Autodesk Fusion 360 part; units mm, degrees
sketch "Sketch1" plane through (0, 0, 0) normal (0, 0, 1) x (1, 0, 0) in component "Hot Plate Mounting Plate"
  line L0 (0, 0) -> (-182, 0) construction
  line L1 (-182, 0) -> (-182, -202) construction
  line L2 (-182, -202) -> (0, -202) construction
  line L3 (0, -202) -> (0, 0) construction
  line L4 (-91, -202) -> (-91, 0) construction
  line L5 (0, -101) -> (-182, -101) construction
  line L6 (-91, 0) -> (-13, 0)
  line L7 (-91, 0) -> (-169, 0)
  line L8 (-91, -202) -> (-13, -202)
  line L9 (-91, -202) -> (-169, -202)
  line L10 (0, -101) -> (0, -13)
  line L11 (0, -101) -> (0, -189)
  line L12 (-182, -101) -> (-182, -189)
  line L13 (-182, -101) -> (-182, -13)
  line L14 (-182, -13) -> (0, -13) construction
  line L15 (0, -189) -> (-182, -189) construction
  line L16 (-13, -202) -> (-13, 0) construction
  line L17 (-169, 0) -> (-169, -202) construction
  line L18 (0, -189) -> (-13, -189)
  line L19 (-13, -202) -> (-13, -189)
  line L20 (-169, -202) -> (-169, -189)
  line L21 (-182, -189) -> (-169, -189)
  line L22 (0, -13) -> (-13, -13)
  line L23 (-13, 0) -> (-13, -13)
  line L24 (-169, 0) -> (-169, -13)
  line L25 (-182, -13) -> (-169, -13)
  dimension "d1" = 182
  dimension "d2" = 202
  dimension "d3" = 78
  dimension "d4" = 78
  dimension "d5" = 78
  dimension "d6" = 78
  dimension "d7" = 88
  dimension "d8" = 88
  dimension "d9" = 88
  dimension "d10" = 88
extrude "Extrude1" add sketch "Sketch1" along normal blind 1 in component "Hot Plate Mounting Plate"
sketch "Sketch3" plane through (0, 0, 1) normal (0, 0, 1) x (-1, 0, 0) in component "Hot Plate Mounting Plate"
  line L0 (182, 13) -> (182, 189)
  line L1 (182, 189) -> (169, 189)
  line L2 (169, 189) -> (169, 202)
  line L3 (169, 202) -> (13, 202)
  line L4 (13, 202) -> (13, 189)
  line L5 (13, 189) -> (0, 189)
  line L6 (0, 189) -> (0, 13)
  line L7 (0, 13) -> (13, 13)
  line L8 (13, 13) -> (13, 0)
  line L9 (13, 0) -> (169, 0)
  line L10 (169, 0) -> (169, 13)
  line L11 (169, 13) -> (182, 13)
  line L12 (177, 13) -> (177, 189) construction
  line L13 (169, 5) -> (13, 5) construction
  line L14 (5, 13) -> (5, 189) construction
  line L15 (13, 197) -> (169, 197) construction
  line L16 (182, 36) -> (0, 36) construction
  line L17 (182, 166) -> (0, 166) construction
  line L18 (146, 0) -> (146, 202) construction
  line L19 (36, 0) -> (36, 202) construction
  circle A0 centre (146, 5) radius 1.75
  circle A1 centre (177, 36) radius 1.75
  circle A2 centre (177, 166) radius 1.75
  circle A3 centre (36, 197) radius 1.75
  circle A4 centre (5, 166) radius 1.75
  circle A5 centre (5, 36) radius 1.75
  circle A6 centre (36, 5) radius 1.75
  line L20 (161, 202) -> (161, 0) construction
  circle A7 centre (161, 197) radius 1.75
  dimension "d44" = 5
  dimension "d45" = 5
  dimension "d46" = 5
  dimension "d47" = 5
  dimension "d48" = 23
  dimension "d49" = 23
  dimension "d50" = 23
  dimension "d51" = 23
  dimension "d52" = 3.5
  dimension "d53" = 3.5
  dimension "d54" = 3.5
  dimension "d56" = 3.5
  dimension "d57" = 3.5
  dimension "d60" = 3.5
  dimension "d61" = 3.5
  dimension "d62" = 8
  dimension "d63" = 3.5
extrude "Extrude3" cut sketch "Sketch3" against normal up to surface (1 mm away) contours A0 | A1 | A2 | A3 | A4 | A5 | A6 | A7 in component "Hot Plate Mounting Plate"
sketch "Sketch4" plane through (0, 0, 1) normal (0, 0, 1) x (-1, 0, 0) in component "Hot Plate Mounting Plate"
  circle A0 centre (5, 36) radius 1.75
  circle A1 centre (5, 166) radius 1.75
  circle A2 centre (177, 166) radius 1.75
  circle A3 centre (36, 5) radius 1.75
  circle A4 centre (146, 5) radius 1.75
  circle A5 centre (36, 197) radius 1.75
  circle A6 centre (177, 36) radius 1.75
  circle A7 centre (161, 197) radius 1.75
  line L0 (182, 13) -> (182, 189)
  line L1 (182, 189) -> (169, 189)
  line L2 (169, 189) -> (169, 202)
  line L3 (169, 202) -> (13, 202)
  line L4 (13, 202) -> (13, 189)
  line L5 (13, 189) -> (0, 189)
  line L6 (0, 189) -> (0, 13)
  line L7 (0, 13) -> (13, 13)
  line L8 (13, 13) -> (13, 0)
  line L9 (13, 0) -> (169, 0)
  line L10 (169, 0) -> (169, 13)
  line L11 (169, 13) -> (182, 13)
  line L12 (182, 101) -> (0, 101) construction
  line L13 (91, 0) -> (91, 202) construction
  line L14 (31, 31) -> (151, 31) construction
  line L15 (151, 31) -> (151, 171) construction
  line L16 (151, 171) -> (31, 171) construction
  line L17 (31, 171) -> (31, 31) construction
  line L18 (31, 31) -> (151, 171) construction
  line L19 (151, 31) -> (31, 171) construction
  line L20 (146, 31) -> (146, 171) construction
  line L21 (151, 36) -> (31, 36) construction
  line L22 (36, 31) -> (36, 171) construction
  line L23 (151, 166) -> (31, 166) construction
  circle A8 centre (146, 36) radius 1.75
  line L24 (151, 96) -> (31, 96) construction
  line L25 (151, 106) -> (31, 106) construction
  circle A9 centre (146, 96) radius 1.75
  circle A10 centre (36, 96) radius 1.75
  circle A11 centre (146, 106) radius 1.75
  circle A12 centre (36, 106) radius 1.75
  circle A13 centre (146, 166) radius 1.75
  circle A14 centre (36, 166) radius 1.75
  circle A15 centre (36, 36) radius 1.75
  line L26 (151, 66) -> (31, 66) construction
  line L27 (151, 136) -> (31, 136) construction
  line L28 (141, 31) -> (141, 171) construction
  circle A16 centre (141, 66) radius 5
  circle A17 centre (141, 136) radius 5
  point P0 (91, 101)
  dimension "d64" = 120
  dimension "d65" = 140
  dimension "d66" = 5
  dimension "d67" = 5
  dimension "d68" = 5
  dimension "d69" = 5
  dimension "d70" = 3.5
  dimension "d71" = 5
  dimension "d72" = 5
  dimension "d73" = 3.5
  dimension "d74" = 3.5
  dimension "d75" = 3.5
  dimension "d76" = 3.5
  dimension "d77" = 3.5
  dimension "d78" = 3.5
  dimension "d79" = 3.5
  dimension "d83" = 35
  dimension "d84" = 35
  dimension "d85" = 10
  dimension "d86" = 10
  dimension "d87" = 10
extrude "Extrude4" cut sketch "Sketch4" against normal up to surface (1 mm away) contours A8 | A9 | A10 | A11 | A12 | A13 | A14 | A15 | A16 | A17 in component "Hot Plate Mounting Plate"
component "Hot Plate Mounting Plate" placed x (1, 0, 0) y (0, 1, 0) z (0, 0, 1) at (0, 0, 0)
Model file for the job. Use its own axes, mm. Coordinates: 2 decimals unless noted, no trailing zeros. Order: outer loops, then holes, each group sorted by start corner. A loop starts at its lowest first (then second) coordinate and runs counter-clockwise, first axis right, second up. Notation, with made-up numbers: (37, 84.5) -> (49, 84.5) arc R37 ccw to (49, 123.5) -> close; hole circle Ø9 at (69.25, 79.5). An arc over 180 degrees is marked (long way). Return JSON: item names as keys, results as strings.
Item 1: Mould opens along X. For faces 1 (the face through (-139.92, -131.12, 0.51)), 2 (the face through (-137.315, -69.379, 0.507)), 3 (the face through (-92, -100, 0)) say: pulls with the +X half, pulls with the -X half, needs draft (parallel to the pull), parting line crosses it, or undercut.
Model answer:
{"face 1": "undercut", "face 2": "undercut", "face 3": "needs draft"}
Item 2: Wall check: line 1 along X through (y, z) = (-5, 0.35); line 2 along X through (y, z) = (-166, 0.35); line 3 along X through (y, z) = (-197, 0.65). Give the ranges that are in metal, low to high. Write a range as from..to.
Model answer:
{"line 1": "x = -169..-147.75, -144.25..-37.75, -34.25..-13", "line 2": "x = -182..-178.75, -175.25..-147.75, -144.25..-37.75, -34.25..-6.75, -3.25..0", "line 3": "x = -169..-162.75, -159.25..-37.75, -34.25..-13"}
Item 3: Slice it at B-B (z = 0.7). Count the separate pieces of the cut face and the enclosed holes in it, then the cut area to 3 significant figures.
Model answer:
{"separate pieces": "1", "enclosed holes": "18", "area": "35,800 mm²"}
Item 4: Pin check, flat tip, straight feed: P1, Ø3, axis at x = -146, y = -36, coming from the +Z side. Stop position of the tip, or through.
Model answer:
{"P1": "passes through"}
Item 5: Slice it at A-A (y = -66). Write the cut outline in (x, z), then the cut area to 3 significant figures.
Model answer:
{"outline": "(-182, 0) -> (-146, 0) -> (-146, 1) -> (-182, 1) -> close; (-136, 0) -> (0, 0) -> (0, 1) -> (-136, 1) -> close", "area": "172 mm²"}
